```python
from build123d import *

# Parameters (mm, degrees)
BOSS_EXTRU_1_DEPTH           = 5
ESQUISSE14_W                 = 99.024162062
ESQUISSE14_H                 = 34
ENL_V_MAT_EXTRU_3_DEPTH      = 10
ESQUISSE15_W                 = 4
ESQUISSE15_H                 = 55
BOSS_EXTRU_2_DEPTH           = 8
ESQUISSE16_W                 = 4
ESQUISSE16_H                 = 55
BOSS_EXTRU_3_DEPTH           = 4
ESQUISSE17_W                 = 4
ESQUISSE17_H                 = 55
BOSS_EXTRU_4_DEPTH           = 4
ESQUISSE18_R                 = 5
BOSS_EXTRU_5_DEPTH           = 5
BOSS_EXTRU_5_DRAFT           = 25
BOSS_EXTRU_5_PROFILE_2_DEPTH = 5
BOSS_EXTRU_5_PROFILE_2_DRAFT = 25
BOSS_EXTRU_5_PROFILE_3_DEPTH = 5
BOSS_EXTRU_5_PROFILE_3_DRAFT = 25
ESQUISSE19_R                 = 9
ENL_V_MAT_EXTRU_4_DEPTH      = 5


with BuildPart() as part:
    # Esquisse3 → Boss.-Extru.1 (new body)
    with BuildSketch(Plane.XY):
        with BuildLine():
            ThreePointArc((75.594209632, 441.104915907), (0.107839882, 447.535495506), (-75.381620177, 441.141295626))
            ThreePointArc((-75.381620177, 441.141295626), (-101.972084627, 403.590452402), (-64.421241404, 376.999987952))
            ThreePointArc((-64.421241404, 376.999987952), (0.092160118, 382.464480398), (64.602920658, 376.968897791))
            ThreePointArc((64.602920658, 376.968897791), (102.166574203, 403.541262362), (75.594209632, 441.104915907))
        make_face()
    extrude(amount=BOSS_EXTRU_1_DEPTH)

    # Esquisse14 → Enlèv. mat.-Extru.3 (cut)
    with BuildSketch(Plane(origin=(0, 0, 0), x_dir=(-1, 0, 0), z_dir=(0, 0, -1))):
        with Locations((-0.090839627, 430.535495506)):
            Rectangle(ESQUISSE14_W, ESQUISSE14_H)
    extrude(amount=-ENL_V_MAT_EXTRU_3_DEPTH, mode=Mode.SUBTRACT)


with BuildPart() as body_2:
    # of the pieces the cut leaves, the one that is kept (enl_v_mat_extru_3_keep)
    add(part.part.solids().sort_by_distance((64.602920658, 376.968897791, 0))[0])

    # Esquisse15 → Boss.-Extru.2 (add)
    with BuildSketch(Plane(origin=(0, 0, 0), x_dir=(-1, 0, 0), z_dir=(0, 0, -1))):
        with Locations((-51.602920658, 411.035495506)):
            Rectangle(ESQUISSE15_W, ESQUISSE15_H)
        with Locations((51.421241404, 411.035495506)):
            Rectangle(ESQUISSE15_W, ESQUISSE15_H)
    extrude(amount=BOSS_EXTRU_2_DEPTH)

    # Esquisse16 → Boss.-Extru.3 (add)
    with BuildSketch(Plane.ZY.offset(-49.602920658)):
        with Locations((-6, 411.035495506)):
            Rectangle(ESQUISSE16_W, ESQUISSE16_H)
    extrude(amount=BOSS_EXTRU_3_DEPTH)

    # Esquisse17 → Boss.-Extru.4 (add)
    with BuildSketch(Plane(origin=(-49.421241404, 0, 0), x_dir=(0, 0, -1), z_dir=(1, 0, 0))):
        with Locations((6, 411.035495506)):
            Rectangle(ESQUISSE17_W, ESQUISSE17_H)
    extrude(amount=BOSS_EXTRU_4_DEPTH)


with BuildPart() as boss_extru_5_tool:
    # Esquisse18 → Boss.-Extru.5 (with draft: the straight prism first)
    with BuildSketch(Plane(origin=(0, 0, 0), x_dir=(-1, 0, 0), z_dir=(0, 0, -1))):
        with Locations((63.421241404, 400.070641789)):
            Circle(ESQUISSE18_R)
    extrude(amount=BOSS_EXTRU_5_DEPTH)
    # Boss.-Extru.5: the draft: its side faces are tilted about the plane it starts from
    boss_extru_5_sides = [boss_extru_5_tool.faces().sort_by_distance(p)[0] for p in [
        (-58.421241404, 400.070641789, -2.5),
    ]]
    draft(boss_extru_5_sides, Plane(origin=(0, 0, 0), x_dir=(-1, 0, 0), z_dir=(0, 0, -1)), BOSS_EXTRU_5_DRAFT)


with BuildPart() as body_2_1:
    add(body_2.part)

    # Boss.-Extru.5: add boss_extru_5_tool
    add(boss_extru_5_tool.part)


with BuildPart() as boss_extru_5_profile_2_tool:
    # Esquisse18 → Boss.-Extru.5 profile 2 (with draft: the straight prism first)
    with BuildSketch(Plane(origin=(0, 0, 0), x_dir=(-1, 0, 0), z_dir=(0, 0, -1))):
        with Locations((84.421241404, 400.070641789)):
            Circle(ESQUISSE18_R)
    extrude(amount=BOSS_EXTRU_5_PROFILE_2_DEPTH)
    # Boss.-Extru.5 profile 2: the draft: its side faces are tilted about the plane it starts from
    boss_extru_5_profile_2_sides = [boss_extru_5_profile_2_tool.faces().sort_by_distance(p)[0] for p in [
        (-79.421241404, 400.070641789, -2.5),
    ]]
    draft(boss_extru_5_profile_2_sides, Plane(origin=(0, 0, 0), x_dir=(-1, 0, 0), z_dir=(0, 0, -1)), BOSS_EXTRU_5_PROFILE_2_DRAFT)


with BuildPart() as body_2_2:
    add(body_2_1.part)

    # Boss.-Extru.5 profile 2: add boss_extru_5_profile_2_tool
    add(boss_extru_5_profile_2_tool.part)


with BuildPart() as boss_extru_5_profile_3_tool:
    # Esquisse18 → Boss.-Extru.5 profile 3 (with draft: the straight prism first)
    with BuildSketch(Plane(origin=(0, 0, 0), x_dir=(-1, 0, 0), z_dir=(0, 0, -1))):
        with Locations((73.921241404, 429.238260821)):
            Circle(ESQUISSE18_R)
    extrude(amount=BOSS_EXTRU_5_PROFILE_3_DEPTH)
    # Boss.-Extru.5 profile 3: the draft: its side faces are tilted about the plane it starts from
    boss_extru_5_profile_3_sides = [boss_extru_5_profile_3_tool.faces().sort_by_distance(p)[0] for p in [
        (-68.921241404, 429.238260821, -2.5),
    ]]
    draft(boss_extru_5_profile_3_sides, Plane(origin=(0, 0, 0), x_dir=(-1, 0, 0), z_dir=(0, 0, -1)), BOSS_EXTRU_5_PROFILE_3_DRAFT)


with BuildPart() as body_2_3:
    add(body_2_2.part)

    # Boss.-Extru.5 profile 3: add boss_extru_5_profile_3_tool
    add(boss_extru_5_profile_3_tool.part)

    # Esquisse19 → Enlèv. mat.-Extru.4 (cut)
    with BuildSketch(Plane(origin=(0, 0, 0), x_dir=(-1, 0, 0), z_dir=(0, 0, -1))):
        with Locations((73.921241404, 409.238260821)):
            Circle(ESQUISSE19_R)
    extrude(amount=-ENL_V_MAT_EXTRU_4_DEPTH, mode=Mode.SUBTRACT)


solid = body_2_3.part
```
Could you check a few things on this model? Use its own coordinates, in mm. A direction names the side the tool comes from. Coordinates: 2 decimals unless noted, no trailing zeros. Write each loop counter-clockwise with the first axis right and the second up, starting at its lowest first coordinate (ties: lowest second). Pieces come first, ordered by that corner, then holes. Notation, with made-up numbers: (43, 87.25) -> (94, 87.25) arc R25 ccw to (94, 123.25) -> close; hole circle Ø6 at (3.5, 52). An arc over 180 degrees is marked (long way). One line per question, with ' | ' between items. Start each with the question number.
1. For faces 4 (the face through (-50, 438.535, -5)), 5 (the face through (49.603, 421, 0)), 6 (the face through (-45.421, 411, -6)), which set-ups out of +Z, -Z, +X, -X, +Y, -Y let a thin tool reach every point of the face, with its end or its side?
2. Will these pins go through, and if not, where does the flat tip stop? P1, Ø7, axis at y = 399.5, z = 0, coming from the -X side; P2, Ø4, axis at x = 68.5, z = 0.5, coming from the +Y side; P3, Ø3, axis at y = 390, z = -6, coming from the -X side; P4, Ø2.5, axis at x = -47.5, z = -2.5, coming from the +Y side.
3. Thinking about a two-plate mould opening in Y: for faces 1 (the face through (-72.75, 418.16, 2.46)), 2 (the face through (-64.839, 397.344, -4.132)), 3 (the face through (-53.421, 411, -4)), which applies, pulls with the +Y half, pulls with the -Y half, needs draft (parallel to the pull), parting line crosses it, or undercut?
4. If we section it at A-A (z = -2): Please give me the cut outline in (x, y).
5. If we section it at B-B (x = 3): Please give me the cut outline in (y, z), and give its area (3 significant figures).
6. If we section it at C-C (x = 31.5): Please give me the cut outline in (y, z), and give its area (3 significant figures).
7. Please list where these lines run through material, in increasing order: line 1 along X through (y, z) = (424.5, -5.75); line 2 along X through (y, z) = (415.5, -0.5); line 3 along X through (y, z) = (427, -0.5).
Return value:
1) face 4: -Z, +X, -X, +Y | face 5: +Y | face 6: -Z, +Y, -Y
2) P1: stops at x = -101.87 | P2: stops at y = 442.57 | P3: stops at x = -53.42 | P4: passes through
3) face 1: undercut | face 2: parting line crosses it | face 3: needs draft
4) outline: circle Ø8.13 at (-84.42, 400.07); circle Ø8.13 at (-73.92, 429.24); circle Ø8.13 at (-63.42, 400.07); (-53.42, 383.54) -> (-49.42, 383.54) -> (-49.42, 438.54) -> (-53.42, 438.54) -> close; (49.6, 383.54) -> (53.6, 383.54) -> (53.6, 438.54) -> (49.6, 438.54) -> close
5) outline: (382.45, 0) -> (413.54, 0) -> (413.54, 5) -> (382.45, 5) -> close | area: 155 mm²
6) outline: (381.17, 0) -> (413.54, 0) -> (413.54, 5) -> (381.17, 5) -> close | area: 162 mm²
7) line 1: x = -53.42 to -45.42, 45.6 to 53.6 | line 2: x = -53.42 to -49.42, 49.6 to 53.6 | line 3: x = -78.13 to -69.71, -53.42 to -49.42, 49.6 to 53.6
